Geometry: final body of the model. Coordinates: model frame, mm. Face numbers are marked on the shaded views. Round coordinates to 2 decimals unless told otherwise and drop trailing zeros. Write each loop counter-clockwise with the first axis right and the second up, starting at its lowest first coordinate (ties: lowest second). Pieces come first, ordered by that corner, then holes. Notation, with made-up numbers: M 67,12.5 L 123,12.5 A26 cw 123,33.5 Z; hole C 54.5,7 d1. An arc over 180 degrees is marked long. Use one line per item in the form item = value. Start each with the question number.
Item 1: Section query A-A (z = 0). Return loops of the section in (x, y), and give its area (3 significant figures).
Item 2: Pull-direction query (Y, two-part tool) for the marked faces 1, 2 and 3; classes: pulls with the +Y half, pulls with the -Y half, needs draft (parallel to the pull), parting line crosses it, or undercut.
Item 3: Ray query, probe 1 along Z at (x, y) = (235, 304); probe 2 along X at (y, z) = (68.5, 46); probe 3 along Z at (x, y) = (205, 338.5). Return the intervals inside material, ascending.
Item 4: Pin query (flat end, axial travel): pin 1 Ø6 at (y, z) = (263.5, -46.5) entering from -X; pin 2 Ø6 at (y, z) = (328.5, 19.5) entering from +X; pin 3 Ø6 at (y, z) = (96.5, 21) entering from -X. Return the tip coordinate at first contact, or that it passes through.
Item 5: Section query C-C (z = -22). Return loops of the section in (x, y), and give its area (3 significant figures).
Item 6: Section query B-B (x = 229). Return loops of the section in (y, z), and give its area (3 significant figures).
from build123d import *

# Parameters (mm, degrees)
F0_R = 76.2
F3_T = -6.35


with BuildPart() as f2:
    # F2: sweep along a path in F1
    with BuildLine(Plane.XY) as f2_path:
        Line((0, 0), (0, 152.4))
        ThreePointArc((0, 152.4), (44.6369265472, 260.1630734528), (152.4, 304.8))
        Line((152.4, 304.8), (304.8, 304.8))
    # F0 (on Front) → F2 (sweep)
    with BuildSketch(Plane.XZ):
        Circle(F0_R)
    sweep(path=f2_path.line)

    # F3
    f3_openings = [f2.faces().sort_by_distance(p)[0] for p in [
        (0, 0, 0),
        (304.8, 304.8, 0),
    ]]
    offset(amount=F3_T, openings=f3_openings)


solid = f2.part
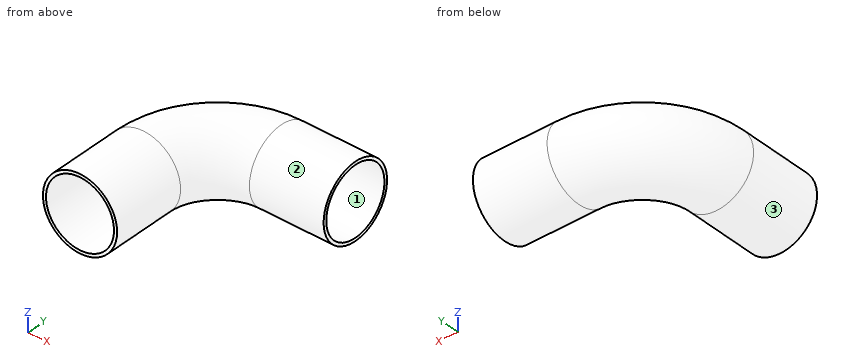
Working result:
q1.outline = M -76.2,0 L -69.85,0 L -69.85,152.4 A222.25 cw 152.4,374.65 L 304.8,374.65 L 304.8,381 L 152.4,381 A228.6 ccw -76.2,152.4 Z; M 69.85,0 L 76.2,0 L 76.2,152.4 A76.2 cw 152.4,228.6 L 304.8,228.6 L 304.8,234.95 L 152.4,234.95 A82.55 ccw 69.85,152.4 Z
q1.area = 6,910 mm²
q2.face_1 = undercut
q2.face_2 = parting line crosses it
q2.face_3 = needs draft
q3.probe_1 = -76.2 to -69.85, 69.85 to 76.2
q3.probe_2 = -60.75 to -52.56, 52.56 to 60.75
q3.probe_3 = -68.34 to -61.18, 61.18 to 68.34
q4.pin_1 = -32.21
q4.pin_2 = 25.82
q4.pin_3 = -74.04
q5.outline = M -72.96,0 L -66.29,0 L -66.29,152.4 A218.69 cw 152.4,371.09 L 304.8,371.09 L 304.8,377.76 L 152.4,377.76 A225.36 ccw -72.96,152.4 Z; M 66.29,0 L 72.96,0 L 72.96,152.4 A79.44 cw 152.4,231.84 L 304.8,231.84 L 304.8,238.51 L 152.4,238.51 A86.11 ccw 66.29,152.4 Z
q5.area = 7,250 mm²
q6.outline = C 304.8,0 d152.4; hole C 304.8,0 d139.7
q6.area = 2,910 mm²
